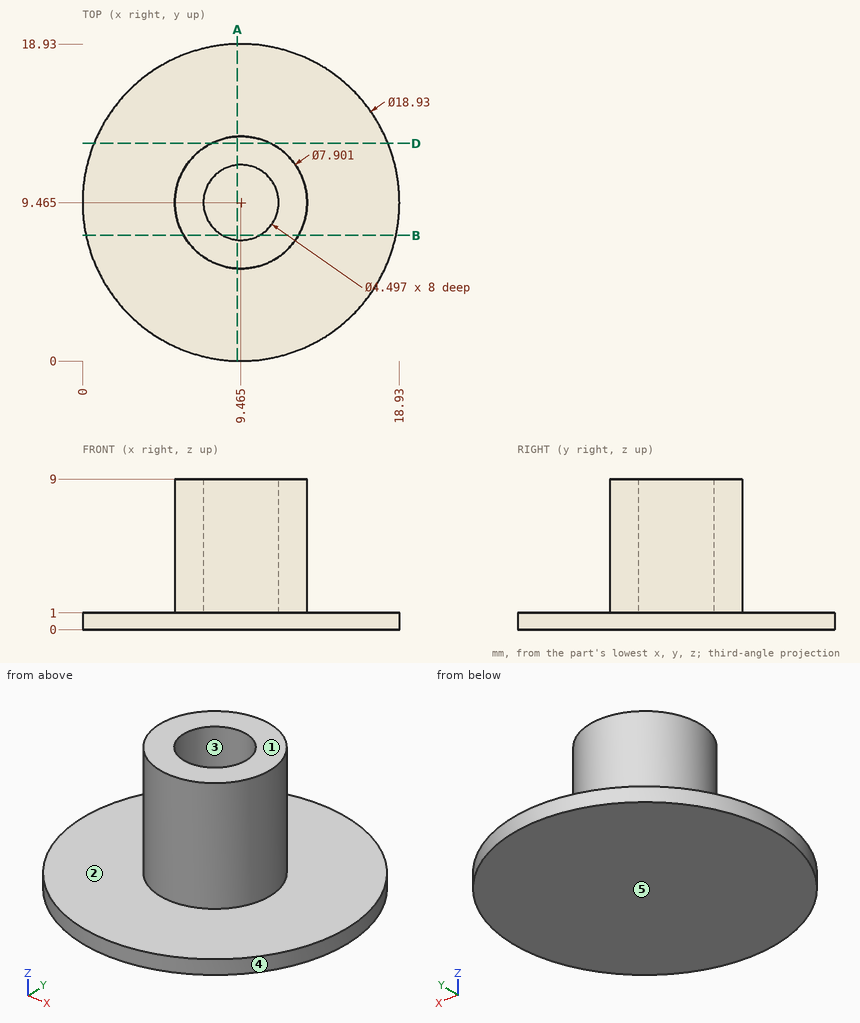
Can you work these out from the drawing? Everything is in mm from the part's minimum corner. A direction names the side the tool comes from. Round coordinates to 2 decimals unless told otherwise and drop trailing zeros. Write each loop counter-clockwise with the first axis right and the second up, starting at its lowest first coordinate (ties: lowest second). Pieces come first, ordered by that corner, then holes. Notation, with made-up numbers: (-19.75, -22) - (13.25, -22) arc R17 cw to (13.25, 3) - close; hole circle Ø2 at (55, 37). An arc over 180 degrees is marked (long way). Use a Markdown table: item, result.
Q1. For pin 1 (4 mm diameter, centred on x = 7, z = 8, fed in from -Y); pin 2 (2.5 mm diameter, centred on x = 9.47, y = 9.47, fed in from +Z); pin 3 (4 mm diameter, centred on y = 2.5, z = 6.5, fed in from -X); pin 4 (5 mm diameter, centred on y = 4.5, z = 3, fed in from +X), each with a flat end and sliding along its axis, tell me the tip position at first contact or that it passes through.
Output values:
| item | result |
|---|---|
| pin 1 | y = 5.54 |
| pin 2 | z = 1 |
| pin 3 | through |
| pin 4 | x = 18.27 |
Q2. I want a section at D-D (y = 13). List the corners of the cut face in (x, z) for me (1 decimal).
Output values:
| item | result |
|---|---|
| outline | (0.7, 0) - (18.2, 0) - (18.2, 1) - (11.2, 1) - (11.2, 9) - (7.7, 9) - (7.7, 1) - (0.7, 1) - close |
Q3. Please list where these lines run through material, in increasing order: L1, parallel to Z at x = 7, y = 17.5; L2, parallel to Y at x = 8.5, z = 3.25 (1 decimal); L3, parallel to Y at x = 8, z = 6.25 (1 decimal).
Output values:
| item | result |
|---|---|
| L1 | 0 to 1 |
| L2 | 5.6 to 7.4, 11.5 to 13.3 |
| L3 | 5.8 to 7.8, 11.2 to 13.1 |
Q4. I want a section at B-B (y = 7.5). List the corners of the cut face in (x, z) for me (1 decimal).
Output values:
| item | result |
|---|---|
| outline | (0.2, 0) - (18.7, 0) - (18.7, 1) - (12.9, 1) - (12.9, 9) - (10.6, 9) - (10.6, 1) - (8.4, 1) - (8.4, 9) - (6, 9) - (6, 1) - (0.2, 1) - close |
Q5. I want a section at A-A (x = 9.25). List the corners of the cut face in (y, z) for me.
Output values:
| item | result |
|---|---|
| outline | (0, 0) - (18.93, 0) - (18.93, 1) - (13.41, 1) - (13.41, 9) - (11.7, 9) - (11.7, 1) - (7.23, 1) - (7.23, 9) - (5.52, 9) - (5.52, 1) - (0, 1) - close |
Q6. For the marked faces 1 and 2, which set-ups out of +Z, -Z, +X, -X, +Y, -Y let a thin tool reach every point of the face, with its end or its side?
Output values:
| item | result |
|---|---|
| face 1 | +Z, +X, -X, +Y, -Y |
| face 2 | +Z |
Q7. Thinking about a two-plate mould opening in X: for the marked faces 3, 4 and 5, which applies, released by +X, released by -X, zero draft, split by the parting line, or undercut?
Output values:
| item | result |
|---|---|
| face 3 | undercut |
| face 4 | split by the parting line |
| face 5 | zero draft |
